from build123d import *

# Parameters (mm, degrees)
EXTRUDE_1_DEPTH                 = 15
SHELL_1_T                       = 2.5
SKETCH_5_R                      = 4.191
EXTRUDE_2_DEPTH                 = 2.5
CUT_EXTRUDE_1_REACH             = 53.635
SKETCH_6_R                      = 2.7083489
CUT_EXTRUDE_1_DIRECTION_2_DEPTH = 1
CUT_EXTRUDE_2_DEPTH             = 52.634942496
CUT_EXTRUDE_2_DEPTH_BACK        = 52.634942496
SKETCH_7_R                      = 1.65
SKETCH_8_W                      = 11.3
SKETCH_8_H                      = 11.108258221
CUT_EXTRUDE_3_DEPTH             = 3


with BuildPart() as part:
    # 草图4 → 凸台-拉伸1 (new body)
    with BuildSketch(Plane.XY):
        with BuildLine():
            Line((32.164875784, -18.408833444), (-36.295124216, -18.408833444))
            ThreePointArc((-36.295124216, -18.408833444), (-37.055264006, -18.093973234), (-37.370124216, -17.333833444))
            Line((-37.370124216, -17.333833444), (-37.370124216, 25.606166556))
            ThreePointArc((-37.370124216, 25.606166556), (-37.055264006, 26.366306345), (-36.295124216, 26.681166556))
            Line((-36.295124216, 26.681166556), (32.164875784, 26.681166556))
            ThreePointArc((32.164875784, 26.681166556), (32.925015574, 26.366306345), (33.239875784, 25.606166556))
            Line((33.239875784, 25.606166556), (33.239875784, -17.333833444))
            ThreePointArc((33.239875784, -17.333833444), (32.925015574, -18.093973234), (32.164875784, -18.408833444))
        make_face()
    extrude(amount=-EXTRUDE_1_DEPTH)

    # 抽壳1
    shell_1_openings = [part.faces().sort_by_distance(p)[0] for p in [
        (-2.065124216, 4.136166556, -15),
    ]]
    offset(amount=SHELL_1_T, openings=shell_1_openings, kind=Kind.INTERSECTION)

    # 草图5 → 凸台-拉伸2 (add)
    with BuildSketch(Plane(origin=(0, 0, 0), x_dir=(-1, 0, 0), z_dir=(0, 0, -1))):
        with Locations(Location((-28.796875784, 22.485238556, 0), (0, 0, 180))):
            Circle(SKETCH_5_R)
        with Locations(Location((7.906124216, -5.962761444, 0), (0, 0, 180))):
            Circle(SKETCH_5_R)
    extrude(amount=EXTRUDE_2_DEPTH)

    # 草图6 → 切除-拉伸1 (cut, up to next)
    with BuildSketch(Plane(origin=(0, 0, 0), x_dir=(-1, 0, 0), z_dir=(0, 0, -1)), mode=Mode.PRIVATE) as cut_extrude_1_sk1:
        with Locations(Location((7.906124216, -5.962761444, 0), (0, 0, 180))):
            Circle(SKETCH_6_R)
    cut_extrude_1_tool1 = extrude(cut_extrude_1_sk1.sketch, amount=-CUT_EXTRUDE_1_REACH, mode=Mode.PRIVATE) & part.part
    # 草图6 → 切除-拉伸1 (cut, up to next)
    with BuildSketch(Plane(origin=(0, 0, 0), x_dir=(-1, 0, 0), z_dir=(0, 0, -1)), mode=Mode.PRIVATE) as cut_extrude_1_sk2:
        with Locations(Location((-28.796875784, 22.485238556, 0), (0, 0, 180))):
            Circle(SKETCH_6_R)
    cut_extrude_1_tool2 = extrude(cut_extrude_1_sk2.sketch, amount=-CUT_EXTRUDE_1_REACH, mode=Mode.PRIVATE) & part.part
    add(cut_extrude_1_tool1.solids().sort_by_distance((-7.906124, -5.962761, 0))[0], mode=Mode.SUBTRACT)
    add(cut_extrude_1_tool2.solids().sort_by_distance((28.796876, 22.485239, 0))[0], mode=Mode.SUBTRACT)

    # 草图6 → 切除-拉伸1 direction 2 (cut)
    with BuildSketch(Plane(origin=(0, 0, 0), x_dir=(-1, 0, 0), z_dir=(0, 0, -1))):
        with Locations(Location((7.906124216, -5.962761444, 0), (0, 0, 180))):
            Circle(SKETCH_6_R)
        with Locations(Location((-28.796875784, 22.485238556, 0), (0, 0, 180))):
            Circle(SKETCH_6_R)
    extrude(amount=CUT_EXTRUDE_1_DIRECTION_2_DEPTH, mode=Mode.SUBTRACT)

    # 草图7 → 切除-拉伸2 (cut, two sides: drawn at the far end of the back side and taken through both)
    with BuildSketch(Plane(origin=(0, 0, 0), x_dir=(-1, 0, 0), z_dir=(0, 0, -1)).offset(-CUT_EXTRUDE_2_DEPTH_BACK)):
        with Locations((7.906124216, -5.962761444)):
            Circle(SKETCH_7_R)
        with Locations((-28.796875784, 22.485238556)):
            Circle(SKETCH_7_R)
    extrude(amount=CUT_EXTRUDE_2_DEPTH + CUT_EXTRUDE_2_DEPTH_BACK, mode=Mode.SUBTRACT)

    # 草图8 → 切除-拉伸3 (cut)
    with BuildSketch(Plane.ZY.offset(39.870124216)):
        with Locations((-9.35, 8.830545142)):
            Rectangle(SKETCH_8_W, SKETCH_8_H)
    extrude(amount=-CUT_EXTRUDE_3_DEPTH, mode=Mode.SUBTRACT)


solid = part.part
For this review, take the finished solid that the model builds, in its own axes (mm). A direction names the side the tool comes from. Coordinates: 2 decimals unless noted, no trailing zeros. Loops run counter-clockwise (first coordinate to the right, second up) from the corner with the lowest first, then second, coordinate; pieces in that order, holes last. Notation, with made-up numbers: (39, -17) - (44, -17) arc R29 cw to (44, 4) - close; hole circle Ø2 at (60.5, -15). An arc over 180 degrees is marked (long way). Use a Markdown table: item, result. Add a question column.
Item 1: We need section B-B (y = -13.5). Give the boundary of the cut face in (x, z).
Item 2: We need section D-D (x = -7). Give the boundary of the cut face in (y, z).
Item 3: We need section C-C (z = -13.5). Give the boundary of the cut face in (x, y) (3 decimals).
Item 4: Insertion check: pin 1 Ø3 at (x, y) = (-39, 10) entering from -Z; pin 2 Ø3 at (x, z) = (-38.5, -9) entering from -Y; pin 3 Ø6.5 at (x, y) = (28.5, 23) entering from -Z; pin 4 Ø3 at (x, y) = (-7.91, -5.96) entering from -Z. Each pin has a flat end and moves straight along its axis. Give the tip position at first contact, or say it passes through.
Item 5: Tool access review of faces 4 (the face through (33.24, 4, -7)), 5 (the face through (-39, 9, -3.7)), 6 (the face through (-8, -4, -1)): name each direction out of +Z, -Z, +X, -X, +Y, -Y from which nothing blocks a thin tool from reaching the whole face with its end or side.
Item 6: Mouldability with a two-part tool opening along X and no side actions: class faces 1 (the face through (34.72, -19.834, -6.127)), 2 (the face through (-2, -18.409, -7)), 3 (the face through (1, -20, -15)) as pulls with the +X half, pulls with the -X half, needs draft (parallel to the pull), parting line crosses it, or undercut.
Item 7: For line 1 (X direction, y = 16.5, z = -10.25); line 2 (Y direction, x = 8, z = -8.5); line 3 (Z direction, x = -3, y = 0), list the stretches that pass through material, from the lowest coordinate up.
Item 8: We need section A-A (x = 22.5). Give the boundary of the cut face in (y, z).
Results list:
| question | item | result |
|---|---|---|
| 1 | outline | (-39.87, -15) - (-37.37, -15) - (-37.37, 0) - (33.24, 0) - (33.24, -15) - (35.74, -15) - (35.74, 2.5) - (-39.87, 2.5) - close |
| 2 | outline | (-20.91, -15) - (-18.41, -15) - (-18.41, 0) - (-10.05, 0) - (-10.05, -2.5) - (-7.34, -2.5) - (-7.34, -1) - (-8.52, -1) - (-8.52, 2.5) - (-20.91, 2.5) - close; (-4.58, -2.5) - (-1.87, -2.5) - (-1.87, 0) - (26.68, 0) - (26.68, -15) - (29.18, -15) - (29.18, 2.5) - (-3.41, 2.5) - (-3.41, -1) - (-4.58, -1) - close |
| 3 | outline | (-39.87, -17.334) arc R3.575 ccw to (-36.295, -20.909) - (32.165, -20.909) arc R3.575 ccw to (35.74, -17.334) - (35.74, 25.606) arc R3.575 ccw to (32.165, 29.181) - (-36.295, 29.181) arc R3.575 ccw to (-39.87, 25.606) - (-39.87, 14.385) - (-37.37, 14.385) - (-37.37, 25.606) arc R1.075 cw to (-36.295, 26.681) - (32.165, 26.681) arc R1.075 cw to (33.24, 25.606) - (33.24, -17.334) arc R1.075 cw to (32.165, -18.409) - (-36.295, -18.409) arc R1.075 cw to (-37.37, -17.334) - (-37.37, 3.276) - (-39.87, 3.276) - close |
| 4 | pin 1 | stops at z = -3.7 |
| 4 | pin 2 | stops at y = -20.84 |
| 4 | pin 3 | stops at z = -2.5 |
| 4 | pin 4 | passes through |
| 5 | face 4 | -Z |
| 5 | face 5 | -Z, -X |
| 5 | face 6 | +Z |
| 6 | face 1 | pulls with the +X half |
| 6 | face 2 | undercut |
| 6 | face 3 | needs draft |
| 7 | line 1 | x = -39.87 to -37.37, 33.24 to 35.74 |
| 7 | line 2 | y = -20.91 to -18.41, 26.68 to 29.18 |
| 7 | line 3 | z = 0 to 2.5 |
| 8 | outline | (-20.91, -15) - (-18.41, -15) - (-18.41, 0) - (26.68, 0) - (26.68, -15) - (29.18, -15) - (29.18, 2.5) - (-20.91, 2.5) - close |
